Geometry check sheet. Reference: the model listing, model coordinates, mm. A direction names the side the tool comes from. Round coordinates to 2 decimals unless told otherwise and drop trailing zeros. Write each loop counter-clockwise with the first axis right and the second up, starting at its lowest first coordinate (ties: lowest second). Pieces come first, ordered by that corner, then holes. Notation, with made-up numbers: (19, -7) -> (61, -7) arc R34 cw to (61, 26) -> close; hole circle Ø10 at (41, 25.5). An arc over 180 degrees is marked (long way). One line per question, with ' | ' between items.
Autodesk Inventor part; units mm, degrees
ref_plane "YZ Plane" through (0, 0, 0) normal (1, 0, 0) x (0, 1, 0)
ref_plane "XY Plane" through (0, 0, 0) normal (0, 0, 1) x (1, 0, 0)
sketch "Sketch1" plane through (0, 0, 0) normal (0, 0, 1) x (1, 0, 0)
  line L0 (-25.4, 4.7625) -> (-25.4, 0)
  line L1 (-25.4, 0) -> (25.4, 0)
  line L2 (25.4, 0) -> (25.4, 4.7625)
  line L3 (25.4, 4.7625) -> (-25.4, 0) construction
  line L4 (-25.4, 4.7625) -> (25.4, 0) construction
  line L5 (-7.62, 4.7625) -> (-7.62, 26.9875)
  line L6 (-7.62, 26.9875) -> (-13.589, 26.9875)
  line L7 (-13.589, 26.9875) -> (-13.589, 7.3025)
  line L8 (13.589, 7.3025) -> (13.589, 26.9875)
  line L9 (13.589, 26.9875) -> (7.62, 26.9875)
  line L10 (7.62, 26.9875) -> (7.62, 4.7625)
  line L11 (0, 4.7625) -> (0, 30.1851) construction
  line L12 (-16.129, 4.7625) -> (-25.4, 4.7625)
  line L13 (25.4, 4.7625) -> (16.129, 4.7625)
  line L14 (7.62, 4.7625) -> (-7.62, 4.7625)
  arc A0 (-16.129, 4.7625) -> (-13.589, 7.3025) centre (-16.129, 7.3025) ccw
  arc A1 (13.589, 7.3025) -> (16.129, 4.7625) centre (16.129, 7.3025) ccw
  point P0 (0, 0)
  point P1 (0, 2.3812)
  point P2 (0, 0)
  dimension "d0" = 26.9875
  dimension "d2" = 50.8
  dimension "d3" = 5.969
  dimension "d4" = 15.24
  dimension "d5" = 2.54
  dimension "d6" = 4.7625
extrude "Extrusion1" add sketch "Sketch1" along normal mid plane 25.4
fillet "Fillet1" radius 6.35 8 edges at (-10.6045, 26.9875, 12.7) (10.6045, 26.9875, 12.7) (-10.6045, 26.9875, -12.7) (10.6045, 26.9875, -12.7) (25.4, 2.3813, 12.7) (25.4, 2.3813, -12.7) (-25.4, 2.3813, 12.7) (-25.4, 2.3813, -12.7)
sketch "Sketch2" plane through (-13.589, 7.3025, -12.7) normal (-1, 0, 0) x (0, 0, 1)
  circle A0 centre (12.7, 12.7) radius 3.3655
  line L0 (6.35, -7.3025) -> (19.05, -7.3025)
  point P0 (12.7, -7.3025)
  point P1 (25.4, -2.54)
  point P2 (12.7, -7.3025)
  dimension "d10" = 6.731
  dimension "d11" = 15.24
extrude "Extrusion2" cut sketch "Sketch2" against normal through all
sketch "Sketch3" plane through (-19.05, 0, -12.7) normal (0, -1, 0) x (1, 0, 0)
  line L0 (0, 12.7) -> (38.1, 12.7) construction
  circle A0 centre (0, 12.7) radius 2.0193
  circle A1 centre (38.1, 12.7) radius 2.0193
  point P0 (19.05, 12.7)
  point P1 (19.05, 12.7)
  dimension "d14" = 4.0386
  dimension "d15" = 38.1
hole "Hole1" at (-19.05, 0, 0) at (19.05, 0, 0) direction (0, 1, 0) diameter 3.9624 end through all
ref_plane "Work Plane1" through (-13.589, 20.0025, 0) normal (0, 1, 0) x (1, 0, 0)
properties part number "TTB 4mm Dyneema Cable Pulley Bracket (ELEV-PULLEY-001)" material "Aluminum 6061"
(1) Access from +Z, -Z, +X, -X, +Y, -Y to the whole of each face (thin tool, end or side, straight path). Record for faces 1 (the flat face through (-11, 26.988, 0)), 2 (the flat face through (22, 4.762, 0)), 3 (the flat face through (0, 4.762, 0)), 4 (the flat face through (-13.589, 15, 0)), 5 (the flat face through (0, 4, 12.7)).
Resolved:
face 1: +Z, -Z, +X, -X, +Y | face 2: +Z, -Z, +X, +Y | face 3: +Z, -Z, +Y | face 4: +Z, -Z, -X, +Y | face 5: +Z, +X, -X, +Y, -Y
(2) Sectioned sample at B-B on z = -5.25. Record the cut outline in (x, y), then the cut area to 3 significant figures.
Resolved:
outline: (-25.4, 0) -> (25.4, 0) -> (25.4, 4.76) -> (16.13, 4.76) arc R2.54 cw to (13.59, 7.3) -> (13.59, 26.99) -> (7.62, 26.99) -> (7.62, 4.76) -> (-7.62, 4.76) -> (-7.62, 26.99) -> (-13.59, 26.99) -> (-13.59, 7.3) arc R2.54 cw to (-16.13, 4.76) -> (-25.4, 4.76) -> close | area: 510 mm2
(3) Sectioned sample at C-C on y = 18.5. Record the cut outline in (x, z).
Resolved:
outline: (-13.59, -12.7) -> (-7.62, -12.7) -> (-7.62, -3.01) -> (-13.59, -3.01) -> close; (-13.59, 3.01) -> (-7.62, 3.01) -> (-7.62, 12.7) -> (-13.59, 12.7) -> close; (7.62, -12.7) -> (13.59, -12.7) -> (13.59, -3.01) -> (7.62, -3.01) -> close; (7.62, 3.01) -> (13.59, 3.01) -> (13.59, 12.7) -> (7.62, 12.7) -> close
(4) Material ranges on line 1 (X direction, y = 3.4, z = 0); line 2 (X direction, y = 21.75, z = -7); line 3 (Y direction, x = -9.75, z = 0), recorded low to high.
Resolved:
line 1: x = -25.4 to -21.03, -17.07 to 17.07, 21.03 to 25.4 | line 2: x = -13.59 to -7.62, 7.62 to 13.59 | line 3: y = 0 to 16.64, 23.37 to 26.99
(5) Go/stop test with flat-tipped pins: pin 1 (10 mm diameter, centred on y = 16, z = 0.5, fed in from -X); pin 2 (3 mm diameter, centred on y = 13, z = 8, fed in from +X); pin 3 (1.5 mm diameter, centred on x = -1.5, z = 8, fed in from -Y); pin 4 (10 mm diameter, centred on x = -20.5, z = 5.5, fed in from +Y). Record where each tip stops, or that it passes through.
Resolved:
pin 1: stops at x = -13.59 | pin 2: stops at x = 13.59 | pin 3: stops at y = 0 | pin 4: stops at y = 4.84
(6) Sectioned sample at D-D on z = 0. Count the separate pieces of the cut face and the enclosed holes in it, then the cut area to 3 significant figures.
Resolved:
separate pieces: 5 | enclosed holes: 0 | area: 392 mm2
(7) Draft check along Z on faces 6 (the cylindrical face through (17.086, 2.415, 0.258)), 7 (the flat face through (25.4, 2, 0)), 8 (the cylindrical face through (-23.59, 2.35, -10.79)). Enter one of: +Z half, -Z half, draft (parallel to the pull), parting line (faces both ways), or undercut.
Resolved:
face 6: undercut | face 7: draft | face 8: -Z half
(8) Sectioned sample at A-A on y = 12.5. Record the cut outline in (x, z), then the cut area to 3 significant figures.
Resolved:
outline: (-13.59, -12.7) -> (-7.62, -12.7) -> (-7.62, 12.7) -> (-13.59, 12.7) -> close; (7.62, -12.7) -> (13.59, -12.7) -> (13.59, 12.7) -> (7.62, 12.7) -> close | area: 303 mm2
